from build123d import *

# Parameters (mm, degrees)
SKETCH1_W           = 63.5
SKETCH1_H           = 50.8
BOSS_EXTRUDE1_DEPTH = 127
SKETCH2_R           = 4.7625
SKETCH2_R_2         = 14.2875
SKETCH2_W           = 12.7
SKETCH2_H           = 101.6
CUT_EXTRUDE1_DEPTH  = 468.663597044
SKETCH3_W           = 31.75
SKETCH3_H           = 76.2
CUT_EXTRUDE2_DEPTH  = 63.5
SKETCH2_3_R         = 25.4
SKETCH2_3_R_2       = 14.2875
CUT_EXTRUDE3_DEPTH  = 12.7
CUT_EXTRUDE4_DEPTH  = 69.85
SKETCH5_W           = 31.75
SKETCH5_H           = 76.2
CUT_EXTRUDE6_DEPTH  = 63.246
CUT_EXTRUDE7_DEPTH  = 69.85


with BuildPart() as part:
    # Sketch1 → Boss-Extrude1 (new body)
    with BuildSketch(Plane.XY):
        Polygon((63.5, -381), (63.5, 381), (31.75, 381), (31.75, 330.2), (-31.75, 330.2), (-31.75, 381), (-63.5, 381), (-63.5, -381), align=None)
        with Locations((0, 355.6)):
            Rectangle(SKETCH1_W, SKETCH1_H)
        with Locations((0, 406.4)):
            Rectangle(SKETCH1_W, SKETCH1_H)
    extrude(amount=BOSS_EXTRUDE1_DEPTH)

    # Sketch2 → Cut-Extrude1 (cut, through all)
    with BuildSketch(Plane(origin=(63.5, 0, 0), x_dir=(0, 0, -1), z_dir=(1, 0, 0))):
        with Locations(Location((-95.25, 406.4, 0), (0, 0, 90))):
            Circle(SKETCH2_R)
        with Locations(Location((-31.75, 406.4, 0), (0, 0, 90))):
            Circle(SKETCH2_R)
        with Locations(Location((-63.5, 254, 0), (0, 0, 90))):
            Circle(SKETCH2_R_2)
        with Locations((-63.5, -330.2)):
            Rectangle(SKETCH2_W, SKETCH2_H)
    extrude(amount=-CUT_EXTRUDE1_DEPTH, mode=Mode.SUBTRACT)

    # Sketch3 → Cut-Extrude2 (cut)
    with BuildSketch(Plane(origin=(0, 0, 0), x_dir=(-1, 0, 0), z_dir=(0, 0, -1))):
        with Locations((-15.875, -215.9)):
            Rectangle(SKETCH3_W, SKETCH3_H)
    extrude(amount=-CUT_EXTRUDE2_DEPTH, mode=Mode.SUBTRACT)

    # Sketch2_3 → Cut-Extrude3 (cut)
    with BuildSketch(Plane(origin=(63.5, 0, 0), x_dir=(0, 0, -1), z_dir=(1, 0, 0))):
        with Locations(Location((-63.5, 254, 0), (0, 0, 90))):
            Circle(SKETCH2_3_R)
        with Locations(Location((-63.5, 254, 0), (0, 0, 90))):
            Circle(SKETCH2_3_R_2, mode=Mode.SUBTRACT)
    extrude(amount=-CUT_EXTRUDE3_DEPTH, mode=Mode.SUBTRACT)

    # Sketch4 → Cut-Extrude4 (cut)
    with BuildSketch(Plane(origin=(63.5, 0, 0), x_dir=(0, 0, -1), z_dir=(1, 0, 0))):
        with BuildLine():
            ThreePointArc((-26.9875, -234.95), (-28.382403955, -231.582403955), (-31.75, -230.1875))
            Line((-31.75, -230.1875), (-31.75, -239.7125))
            ThreePointArc((-31.75, -239.7125), (-28.382403955, -238.317596045), (-26.9875, -234.95))
        make_face()
        with BuildLine():
            Line((-31.75, -239.7125), (-31.75, -230.1875))
            ThreePointArc((-31.75, -230.1875), (-36.5125, -234.95), (-31.75, -239.7125))
        make_face()
        with BuildLine():
            ThreePointArc((-26.9875, -196.85), (-28.382403955, -193.482403955), (-31.75, -192.0875))
            Line((-31.75, -192.0875), (-31.75, -201.6125))
            ThreePointArc((-31.75, -201.6125), (-28.382403955, -200.217596045), (-26.9875, -196.85))
        make_face()
        with BuildLine():
            Line((-31.75, -201.6125), (-31.75, -192.0875))
            ThreePointArc((-31.75, -192.0875), (-36.5125, -196.85), (-31.75, -201.6125))
        make_face()
    extrude(amount=-CUT_EXTRUDE4_DEPTH, mode=Mode.SUBTRACT)

    # Sketch5 → Cut-Extrude6 (cut)
    with BuildSketch(Plane.ZY.offset(63.5)):
        with Locations((79.375, -215.9)):
            Rectangle(SKETCH5_W, SKETCH5_H)
    extrude(amount=-CUT_EXTRUDE6_DEPTH, mode=Mode.SUBTRACT)

    # Sketch6 → Cut-Extrude7 (cut)
    with BuildSketch(Plane.XY.offset(127)):
        with BuildLine():
            ThreePointArc((-26.9875, -234.95), (-28.382403955, -231.582403955), (-31.75, -230.1875))
            Line((-31.75, -230.1875), (-31.75, -239.7125))
            ThreePointArc((-31.75, -239.7125), (-28.382403955, -238.317596045), (-26.9875, -234.95))
        make_face()
        with BuildLine():
            Line((-31.75, -239.7125), (-31.75, -230.1875))
            ThreePointArc((-31.75, -230.1875), (-36.5125, -234.95), (-31.75, -239.7125))
        make_face()
        with BuildLine():
            ThreePointArc((-26.9875, -196.85), (-28.382403955, -193.482403955), (-31.75, -192.0875))
            Line((-31.75, -192.0875), (-31.75, -201.6125))
            ThreePointArc((-31.75, -201.6125), (-28.382403955, -200.217596045), (-26.9875, -196.85))
        make_face()
        with BuildLine():
            Line((-31.75, -201.6125), (-31.75, -192.0875))
            ThreePointArc((-31.75, -192.0875), (-36.5125, -196.85), (-31.75, -201.6125))
        make_face()
    extrude(amount=-CUT_EXTRUDE7_DEPTH, mode=Mode.SUBTRACT)


solid = part.part
Geometry: final body of the model. Coordinates: model frame, mm. A direction names the side the tool comes from. Coordinates: 2 decimals unless noted, no trailing zeros. Order: outer loops, then holes, each group sorted by start corner. A loop starts at its lowest first (then second) coordinate and runs counter-clockwise, first axis right, second up. Notation, with made-up numbers: M -29.75,50.5 L 6.25,50.5 A16 cw 6.25,66.5 Z; hole C 70,-9.75 d4. An arc over 180 degrees is marked long. One line per question, with ' | ' between items. Start each with the question number.
Item 1: Draft query along X for faces 5 (the flat face through (16, -177.8, 31)), 6 (the flat face through (0, 431.8, 63)), 7 (the flat face through (-0.254, -215, 79)), 8 (the flat face through (63.5, -5, 63)). Return one class per face: released by +X, released by -X, zero draft, split by the parting line, or undercut.
Item 2: Cut plane B-B, the plane z = 16. Return the cut outline in (x, y).
Item 3: Pin query (flat end, axial travel): pin 1 Ø16 at (x, y) = (14.5, -203) entering from -Z; pin 2 Ø12.5 at (y, z) = (406.4, 95.25) entering from +X; pin 3 Ø3 at (y, z) = (-197, 33) entering from +X. Return the tip coordinate at first contact, or that it passes through.
Item 4: Set-up query: faces 1 (the flat face through (50.8, 265, 53)), 2 (the flat face through (1, -331, 57.15)), 3 (the flat face through (31.75, -216, 31)), 4 (the flat face through (-32, -216, 63.5)). Return all of +Z, -Z, +X, -X, +Y, -Y with unobstructed straight access to the full face (end or side cutting, diameter ignored); none if empty.
Item 5: Cut plane C-C, the plane y = -312. Return the cut outline in (x, z), then the cut area to 3 significant figures.
Item 6: Cut plane A-A, the plane y = 254. Return the cut outline in (x, z).
Item 7: Ray query, probe 1 along Z at (x, y) = (6, 406.4); probe 2 along Y at (x, z) = (16, 31); probe 3 along Z at (x, y) = (-20, 254). Return the intervals inside material, ascending. Write a range as [from, to].
A:
1) face 5: undercut | face 6: zero draft | face 7: released by -X | face 8: released by +X
2) outline: M -63.5,-381 L 63.5,-381 L 63.5,381 L 31.75,381 L 31.75,431.8 L -31.75,431.8 L -31.75,381 L -63.5,381 Z; hole M 0,-254 L 31.75,-254 L 31.75,-177.8 L 0,-177.8 Z
3) pin 1: stops at z = 63.5 | pin 2: stops at x = 31.75 | pin 3: stops at x = -6.35
4) face 1: +X | face 2: +X, -X, -Y | face 3: -Z | face 4: -X
5) outline: M -63.5,0 L 63.5,0 L 63.5,57.15 L -63.5,57.15 Z; M -63.5,69.85 L 63.5,69.85 L 63.5,127 L -63.5,127 Z | area: 14,500 mm2
6) outline: M -63.5,0 L 63.5,0 L 63.5,38.1 L 50.8,38.1 L 50.8,49.21 L -63.5,49.21 Z; M -63.5,77.79 L 50.8,77.79 L 50.8,88.9 L 63.5,88.9 L 63.5,127 L -63.5,127 Z
7) probe 1: z = [0, 26.99], [36.51, 90.49], [100.01, 127] | probe 2: y = [-381, -254], [-177.8, 401.7], [411.1, 431.8] | probe 3: z = [0, 49.21], [77.79, 127]
